Verification items for the finished model (mm, model axes). A direction names the side the tool comes from. Round coordinates to 2 decimals unless told otherwise and drop trailing zeros. Write each loop counter-clockwise with the first axis right and the second up, starting at its lowest first coordinate (ties: lowest second). Pieces come first, ordered by that corner, then holes. Notation, with made-up numbers: (73, 66) - (109, 66) arc R24 cw to (109, 86) - close; hole circle Ø2 at (-24, -18.75). An arc over 180 degrees is marked (long way). Answer as a JSON object with one key per item and string values. Group by question number.
1) Mould release check, pull along Y, two halves, no side actions. Record for faces 1 (the flat face through (-26, 26, 2)), 2 (the flat face through (435, 3, 13)), 3 (the flat face through (436, 50.8, 13)), 4 (the flat face through (422, 31, 0)): +Y half, -Y half, draft (parallel to the pull), parting line (faces both ways), or undercut.
2) Go/stop test with a flat-tipped pin: pin 1 Ø3 at (y, z) = (28, 22) entering from -X. Record where the tip stops, or that it passes through.
3) Thickness scan on line 1 (Z direction, x = 758.4, y = 48.9); line 2 (Y direction, x = 323, z = 4.5); line 3 (Z direction, x = 611, y = 41.5). Record the ranges inside material, lowest first.
4) Set-up check for faces 5 (the flat face through (883.7, 25.3, 2.3)), 6 (the flat face through (436, 30, 3)): record each of +Z, -Z, +X, -X, +Y, -Y from which the full face is reachable in a straight line by a thin tool's end or side.
5) Section check A-A (x = 628.5). Enter the section's corners in (y, z), then the cut area to 3 significant figures.
```python
from build123d import *

# Parameters (mm, degrees)
SKETCH1_R               = 7
BOSS_EXTRUDE1_DEPTH     = 25.4
SKETCH3_W               = 19.4
SKETCH3_H               = 44.8
CUT_EXTRUDE1_DEPTH      = 1046.4
CUT_EXTRUDE1_DEPTH_BACK = 201.4
SKETCH4_R               = 2.5
CUT_EXTRUDE2_DEPTH      = 22
CUT_EXTRUDE2_DEPTH_BACK = 22


with BuildPart() as part:
    # Sketch1 → Boss-Extrude1 (new body)
    with BuildSketch(Plane.XY):
        Polygon((-50.8, 50.8), (0, 0), (858.4, 0), (909.2, 50.8), align=None)
        with Locations((429.2, 26.4)):
            Circle(SKETCH1_R, mode=Mode.SUBTRACT)
    extrude(amount=BOSS_EXTRUDE1_DEPTH)

    # Sketch3 → Cut-Extrude1 (cut, two sides)
    with BuildSketch(Plane(origin=(0, 0, 0), x_dir=(0, 0, -1), z_dir=(1, 0, 0))) as cut_extrude1_sk:
        with Locations((-12.7, 25.4)):
            Rectangle(SKETCH3_W, SKETCH3_H)
    extrude(amount=CUT_EXTRUDE1_DEPTH, mode=Mode.SUBTRACT)
    extrude(cut_extrude1_sk.sketch, amount=-CUT_EXTRUDE1_DEPTH_BACK, mode=Mode.SUBTRACT)

    # Sketch4 → Cut-Extrude2 (cut, two sides)
    with BuildSketch(Plane(origin=(0, 50.8, 0), x_dir=(1, 0, 0), z_dir=(0, 1, 0))) as cut_extrude2_sk:
        with Locations((25, -12.7)):
            Circle(SKETCH4_R)
        with Locations((100, -12.7)):
            Circle(SKETCH4_R)
        with Locations((200, -12.7)):
            Circle(SKETCH4_R)
        with Locations((275, -12.7)):
            Circle(SKETCH4_R)
        with Locations((833.4, -12.7)):
            Circle(SKETCH4_R)
        with Locations((758.4, -12.7)):
            Circle(SKETCH4_R)
        with Locations((658.4, -12.7)):
            Circle(SKETCH4_R)
        with Locations((583.4, -12.7)):
            Circle(SKETCH4_R)
    extrude(amount=CUT_EXTRUDE2_DEPTH, mode=Mode.SUBTRACT)
    extrude(cut_extrude2_sk.sketch, amount=-CUT_EXTRUDE2_DEPTH_BACK, mode=Mode.SUBTRACT)


solid = part.part
```
Returned:
{
 "1": {"face 1": "-Y half", "face 2": "undercut", "face 3": "+Y half", "face 4": "draft"},
 "2": {"pin 1": "x = -29.45"},
 "3": {"line 1": "0 to 10.2, 15.2 to 25.4", "line 2": "0 to 3, 47.8 to 50.8", "line 3": "0 to 3, 22.4 to 25.4"},
 "4": {"face 5": "+Z, -Z, +X, -Y", "face 6": "+X, -X"},
 "5": {"outline": "(0, 0) - (50.8, 0) - (50.8, 25.4) - (0, 25.4) - close; hole (3, 3) - (47.8, 3) - (47.8, 22.4) - (3, 22.4) - close", "area": "421 mm2"}
}
